Geometry check sheet. Reference: drawing and pictorial views, mm from the part's lowest x, y, z. A direction names the side the tool comes from. Coordinates: 2 decimals unless noted, no trailing zeros. Write each loop counter-clockwise with the first axis right and the second up, starting at its lowest first coordinate (ties: lowest second). Pieces come first, ordered by that corner, then holes. Notation, with made-up numbers: (-38, 3) - (-22, 3) arc R19 ccw to (-22, 16) - close; hole circle Ø8 at (-40, 19.5). An arc over 180 degrees is marked (long way). Use one line per item in the form item = value. Start each with the question number.
(1) Sectioned sample at A-A (y = 20.5). Record the cut outline in (x, z), and give its area (3 significant figures).
(2) Mould release check, pull along Y, two halves, no side actions. Record for the marked faces 3, 4 and 5: released by +Y, released by -Y, zero draft, split by the parting line, or undercut.
(3) Sectioned sample at D-D (x = 3.5). Record the cut outline in (y, z), and give its area (3 significant figures).
(4) Sectioned sample at B-B (x = 18.5). Record the cut outline in (y, z).
(5) Sectioned sample at C-C (z = 7.25). Record the cut outline in (x, y) (3 decimals).
(6) Material ranges on line 1 (Y direction, x = 16, z = 3); line 2 (Z direction, x = 11, y = 29.5); line 3 (Y direction, x = 6, z = 0.5), recorded low to high. Write a range as [from, to].
(7) Gauge pin test, flat ends, axial feed: pin 1 Ø5 at (y, z) = (7.5, 4.5) entering from +X; pin 2 Ø6 at (y, z) = (11, 8.5) entering from -X; pin 3 Ø1.5 at (x, z) = (16, 8) entering from -Y (3 decimals); pin 4 Ø10 at (x, y) = (7, 20) entering from +Z. Record the tip position at first contact, or that the pin passes through.
(8) Tool access check on the marked faces 1 and 2. Record the directions out of +Z, -Z, +X, -X, +Y, -Y that give a thin tool (end or side, any length) a straight path to the whole face; none if there is none.
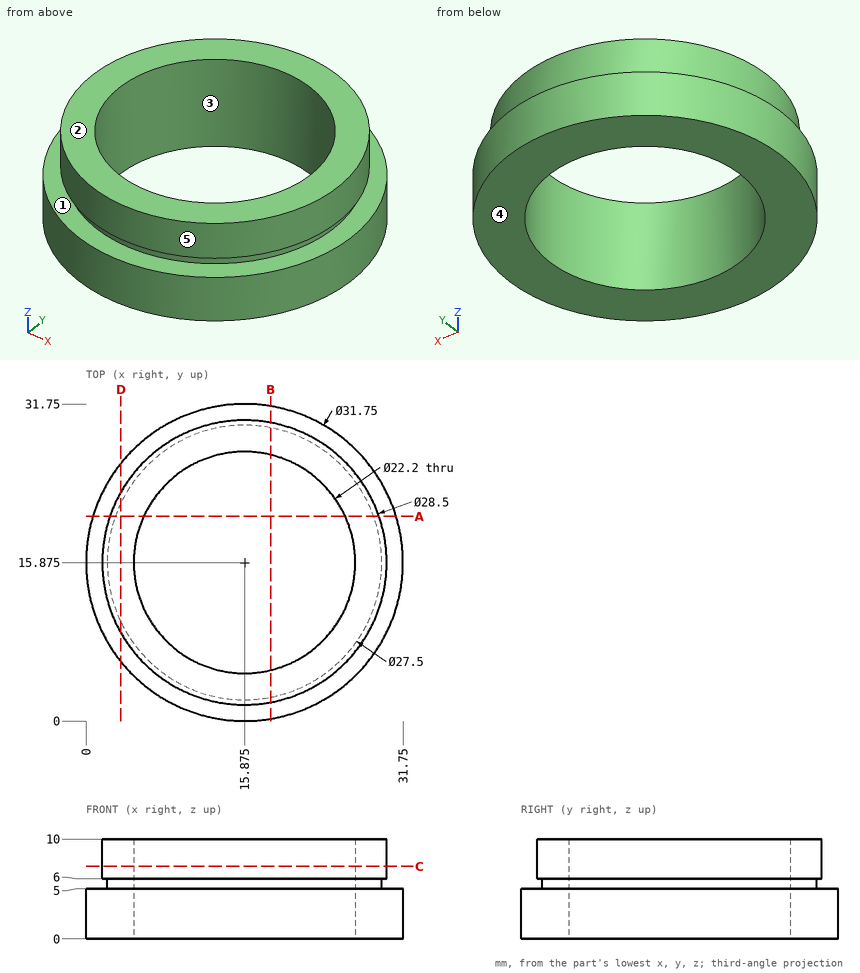
Answers below:
q1.outline = (0.69, 0) - (5.78, 0) - (5.78, 10) - (2.4, 10) - (2.4, 6) - (2.93, 6) - (2.93, 5) - (0.69, 5) - close; (25.97, 0) - (31.06, 0) - (31.06, 5) - (28.82, 5) - (28.82, 6) - (29.35, 6) - (29.35, 10) - (25.97, 10) - close
q1.area = 83.8 mm2
q2.face_3 = undercut
q2.face_4 = zero draft
q2.face_5 = split by the parting line
q3.outline = (5.93, 0) - (25.82, 0) - (25.82, 5) - (21.87, 5) - (21.87, 6) - (22.94, 6) - (22.94, 10) - (8.81, 10) - (8.81, 6) - (9.88, 6) - (9.88, 5) - (5.93, 5) - close
q3.area = 168 mm2
q4.outline = (0.22, 0) - (5.09, 0) - (5.09, 10) - (1.87, 10) - (1.87, 6) - (2.38, 6) - (2.38, 5) - (0.22, 5) - close; (26.66, 0) - (31.53, 0) - (31.53, 5) - (29.37, 5) - (29.37, 6) - (29.88, 6) - (29.88, 10) - (26.66, 10) - close
q5.outline = circle Ø28.5 at (15.875, 15.875); hole circle Ø22.2 at (15.875, 15.875)
q6.line_1 = [0, 4.78], [26.97, 31.75]
q6.line_2 = [0, 5]
q6.line_3 = [3.45, 10.81], [20.94, 28.3]
q7.pin_1 = 30.62
q7.pin_2 = 1.75
q7.pin_3 = 1.625
q7.pin_4 = 10
q8.face_1 = none
q8.face_2 = +Z, +X, -X, +Y, -Y
